```python
from build123d import *

# Parameters (mm, degrees)
BOSS_EXTRUDE1_DEPTH = 25.4
SKETCH3_R           = 4.765
CUT_EXTRUDE1_DEPTH  = 128
SKETCH5_R           = 10.5
CUT_EXTRUDE2_DEPTH  = 10
SKETCH6_W           = 11.049
SKETCH6_H           = 9.53
CUT_EXTRUDE3_DEPTH  = 10


with BuildPart() as part:
    # Sketch2 → Boss-Extrude1 (new body, symmetric)
    with BuildSketch(Plane.XY):
        with BuildLine():
            Line((-15.875, 0), (15.875, 0))
            Line((15.875, 0), (15.875, 127))
            Line((15.875, 127), (12.7, 127))
            ThreePointArc((12.7, 127), (10.45493597, 126.07006403), (9.525, 123.825))
            Line((9.525, 123.825), (9.525, 9.525))
            ThreePointArc((9.525, 9.525), (8.59506403, 7.27993597), (6.35, 6.35))
            Line((6.35, 6.35), (-12.7, 6.35))
            Line((-12.7, 6.35), (-15.875, 6.35))
            Line((-15.875, 6.35), (-15.875, 3.175))
            Line((-15.875, 3.175), (-15.875, 0))
        make_face()
    extrude(amount=BOSS_EXTRUDE1_DEPTH, both=True)

    # Sketch3 → Cut-Extrude1 (cut, through all)
    with BuildSketch(Plane.XZ):
        with Locations((-4.826, 0)):
            Circle(SKETCH3_R)
    extrude(amount=-CUT_EXTRUDE1_DEPTH, mode=Mode.SUBTRACT)

    # Sketch5 → Cut-Extrude2 (cut)
    with BuildSketch(Plane(origin=(15.875, 0, 0), x_dir=(0, 0, -1), z_dir=(1, 0, 0))):
        with Locations((0, 105)):
            Circle(SKETCH5_R)
    extrude(amount=-CUT_EXTRUDE2_DEPTH, mode=Mode.SUBTRACT)

    # Sketch6 → Cut-Extrude3 (cut)
    with BuildSketch(Plane.XZ):
        with Locations((-10.3505, 0)):
            Rectangle(SKETCH6_W, SKETCH6_H)
    extrude(amount=-CUT_EXTRUDE3_DEPTH, mode=Mode.SUBTRACT)


solid = part.part
```
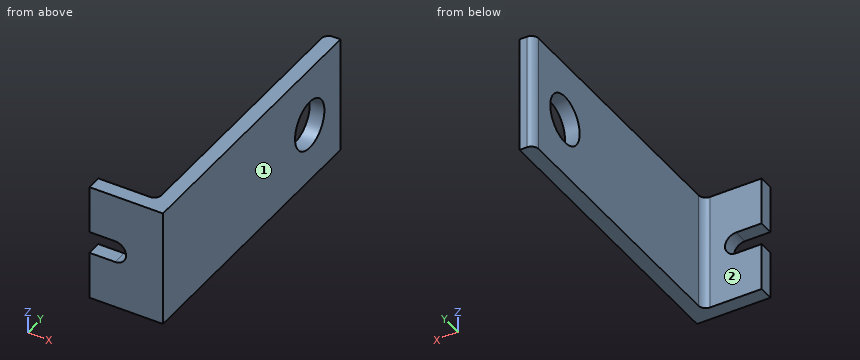
Geometry: final body of the model. Coordinates: model frame, mm. Face numbers are marked on the shaded views. A direction names the side the tool comes from. Round coordinates to 2 decimals unless told otherwise and drop trailing zeros. Loops run counter-clockwise (first coordinate to the right, second up) from the corner with the lowest first, then second, coordinate; pieces in that order, holes last.
Item 1: Section B-B, the plane x = -12.5. Output: boundary loops of the cut face in (y, z) (3 decimals).
Checked values:
outline: (0, -25.4) - (6.35, -25.4) - (6.35, -4.765) - (0, -4.765) - close; (0, 4.765) - (6.35, 4.765) - (6.35, 25.4) - (0, 25.4) - close
Item 2: Section D-D, the plane z = 13. Output: boundary loops of the cut face in (x, y) (3 decimals).
Checked values:
outline: (-15.875, 0) - (15.875, 0) - (15.875, 127) - (12.7, 127) arc R3.175 ccw to (9.525, 123.825) - (9.525, 9.525) arc R3.175 cw to (6.35, 6.35) - (-15.875, 6.35) - close
Item 3: Line query: L1, parallel to Y at x = 14, z = 0; L2, parallel to X at y = 111, z = -11 (3 decimals); L3, parallel to Y at x = -4, z = 7. Output: solid intervals per line, ascending.
Checked values:
L1: y = 0 to 94.5, 115.5 to 127
L2: x = 9.525 to 15.875
L3: y = 0 to 6.35
Item 4: Section A-A, the plane y = 105. Output: boundary loops of the cut face in (x, z) (3 decimals).
Checked values:
outline: (9.525, -25.4) - (15.875, -25.4) - (15.875, -10.5) - (9.525, -10.5) - close; (9.525, 10.5) - (15.875, 10.5) - (15.875, 25.4) - (9.525, 25.4) - close
Item 5: Contact query for flat-ended pins moving along their axis: P1, Ø3, axis at y = 50, z = 5.5, coming from the -X side (3 decimals); P2, Ø6.5, axis at x = 0.5, z = 5.5, coming from the +Y side; P3, Ø2, axis at x = 11.5, z = 6, coming from the +Y side; P4, Ø6, axis at x = -12.5, z = 0.5, coming from the -Y side. Output: stop coordinate, or through.
Checked values:
P1: stops at x = 9.525
P2: stops at y = 6.35
P3: stops at y = 126.99
P4: passes through
Item 6: Section C-C, the plane z = 0. Output: boundary loops of the cut face in (x, y) (3 decimals).
Checked values:
outline: (-0.061, 0) - (15.875, 0) - (15.875, 94.5) - (9.525, 94.5) - (9.525, 9.525) arc R3.175 cw to (6.35, 6.35) - (-0.061, 6.35) - close; (9.525, 115.5) - (15.875, 115.5) - (15.875, 127) - (12.7, 127) arc R3.175 ccw to (9.525, 123.825) - close
Item 7: Reachability of the marked faces 1 and 2 from +Z, -Z, +X, -X, +Y, -Y: full face, straight path, thin tool, end or side. Return the list, or none.
Checked values:
face 1: +Z, -Z, +X, +Y, -Y
face 2: +Z, -Z, -X, +Y
